The listing builds one solid part. Answer for the finished solid, in the listing's coordinates (mm). A direction names the side the tool comes from. Give positions to 0.01 mm unless a question says otherwise; leave off trailing zeros. Loops run counter-clockwise (first coordinate to the right, second up) from the corner with the lowest first, then second, coordinate; pieces in that order, holes last. Notation, with made-up numbers: (51.25, -21.75) - (69.25, -21.75) arc R14 ccw to (69.25, -10.75) - close; hole circle Ø10 at (85, -10). An arc over 180 degrees is marked (long way). Answer as CSV lines item,"result". Start each with the question number.
1) For faces 1 (the face through (15, 10, -16)), 2 (the face through (18, 9.4, -18)), 3 (the face through (-18, 17, 17)), determine the directions among +Z, -Z, +X, -X, +Y, -Y from which every point of the face is accessible in a straight line to the end or side of a thin tool.
2) Flat-ended cylindrical pins translate along their axes: pin 1 (2.5 mm diameter, centred on x = -15.5, z = -15.5, fed in from +Y); pin 2 (7.5 mm diameter, centred on x = -17, z = 17, fed in from +Y); pin 3 (1.6 mm diameter, centred on x = 15.5, z = 16, fed in from -Y); pin 4 (10 mm diameter, centred on x = -14, y = 41, fed in from -Z). Find the tip coordinate at first contact, or state that the pin passes through.
3) A cutting plane is placed at B-B (z = 0). Determine the outline of the cut face in (x, y).
4) A cutting plane is placed at D-D (y = 20). Determine the outline of the cut face in (x, z), and give its area (3 significant figures).
5) For a pull along Z with two mould halves and no side action, classify faces 4 (the face through (0, 17, -21)), 5 (the face through (-18, 24.6, -18)), 6 (the face through (-15, 29.5, -16)), 7 (the face through (-16, 10, -16)) as pulls with the +Z half, pulls with the -Z half, needs draft (parallel to the pull), parting line crosses it, or undercut.
6) A cutting plane is placed at C-C (x = 0). Determine the outline of the cut face in (y, z).
7) A cutting plane is placed at A-A (y = 5). Determine the outline of the cut face in (x, z).
8) Find the intervals of material crossed by line 1 along X through (y, z) = (6, 15.5); line 2 along X through (y, z) = (34.8, 0); line 3 along Z through (x, y) = (-15, 32), in increasing order.
```python
from build123d import *

# Parameters (mm, degrees)
SKETCH4_W               = 42
SKETCH4_H               = 42
BOTTOM_DEPTH            = 9.4
MIDDLE_DEPTH            = 15.2
SKETCH8_W               = 42
SKETCH8_H               = 42
TOP_DEPTH               = 9.4
CHAMFER1_SIZE           = 5
SKETCH9_R               = 11
SKETCH9_R_2             = 3.5
RING_DEPTH              = 2
SKETCH10_R              = 2.5
SHAFT_DEPTH             = 24
CUT_EXTRUDE3_DEPTH      = 5
CUT_EXTRUDE3_DEPTH_BACK = 5
SKETCH11_W              = 2.239647547
SKETCH11_H              = 24.242457261
SKETCH12_R              = 1.55
CUT_EXTRUDE4_DEPTH      = 4.5
CUT_EXTRUDE5_START      = -10
SKETCH15_R              = 1.55
CUT_EXTRUDE5_DEPTH      = 10


with BuildPart() as part:
    # Sketch4 → Bottom (new body)
    with BuildSketch(Plane(origin=(0, 0, 0), x_dir=(1, 0, 0), z_dir=(0, 1, 0))):
        Rectangle(SKETCH4_W, SKETCH4_H)
    extrude(amount=BOTTOM_DEPTH)

    # Sketch6 → Middle (add)
    with BuildSketch(Plane(origin=(0, 9.4, 0), x_dir=(1, 0, 0), z_dir=(0, 1, 0))):
        Polygon((-21, -14), (-14, -21), (14, -21), (21, -14), (21, 14), (14, 21), (-14, 21), (-21, 14), align=None)
    extrude(amount=MIDDLE_DEPTH)

    # Sketch8 → Top (add)
    with BuildSketch(Plane(origin=(0, 24.6, 0), x_dir=(1, 0, 0), z_dir=(0, 1, 0))):
        Rectangle(SKETCH8_W, SKETCH8_H)
    extrude(amount=TOP_DEPTH)

    # Chamfer1
    chamfer1_edges = [part.edges().sort_by_distance(p)[0] for p in [
        (21, 29.3, 21),
        (21, 29.3, -21),
        (-21, 29.3, -21),
        (-21, 29.3, 21),
        (-21, 4.7, 21),
        (-21, 4.7, -21),
        (21, 4.7, -21),
        (21, 4.7, 21),
    ]]
    chamfer(chamfer1_edges, length=CHAMFER1_SIZE)

    # Sketch9 → Ring (add)
    with BuildSketch(Plane(origin=(0, 34, 0), x_dir=(1, 0, 0), z_dir=(0, 1, 0))):
        with Locations(Location((0, 0, 0), (0, 0, 270))):
            Circle(SKETCH9_R)
        with Locations(Location((0, 0, 0), (0, 0, 270))):
            Circle(SKETCH9_R_2, mode=Mode.SUBTRACT)
    extrude(amount=RING_DEPTH)

    # Sketch10 → Shaft (add)
    with BuildSketch(Plane(origin=(0, 34, 0), x_dir=(1, 0, 0), z_dir=(0, 1, 0))):
        with Locations(Location((0, 0, 0), (0, 0, 90))):
            Circle(SKETCH10_R)
    extrude(amount=SHAFT_DEPTH)

    # Sketch11 → Cut-Extrude3 (cut, two sides: drawn at the far end of the back side and taken through both)
    with BuildSketch(Plane(origin=(0, 0, 0), x_dir=(0, 0, -1), z_dir=(1, 0, 0)).offset(-CUT_EXTRUDE3_DEPTH_BACK)):
        with Locations((2.338622492, 61.12122863)):
            Rectangle(SKETCH11_W, SKETCH11_H)
    extrude(amount=CUT_EXTRUDE3_DEPTH + CUT_EXTRUDE3_DEPTH_BACK, mode=Mode.SUBTRACT)

    # Sketch12 → Cut-Extrude4 (cut)
    with BuildSketch(Plane(origin=(0, 34, 0), x_dir=(1, 0, 0), z_dir=(0, 1, 0))):
        with Locations(Location((15.5, -15.5, 0), (0, 0, 270))):
            Circle(SKETCH12_R)
        with Locations(Location((-15.5, -15.5, 0), (0, 0, 270))):
            Circle(SKETCH12_R)
        with Locations(Location((-15.5, 15.5, 0), (0, 0, 270))):
            Circle(SKETCH12_R)
        with Locations(Location((15.5, 15.5, 0), (0, 0, 270))):
            Circle(SKETCH12_R)
    extrude(amount=-CUT_EXTRUDE4_DEPTH, mode=Mode.SUBTRACT)

    # Sketch15 → Cut-Extrude5 (cut)
    with BuildSketch(Plane.XZ.offset(CUT_EXTRUDE5_START)):
        with Locations(Location((15.5, 15.5, 0), (0, 0, 90))):
            Circle(SKETCH15_R)
        with Locations(Location((15.5, -15.5, 0), (0, 0, 90))):
            Circle(SKETCH15_R)
        with Locations(Location((-15.5, 15.5, 0), (0, 0, 90))):
            Circle(SKETCH15_R)
        with Locations(Location((-15.5, -15.5, 0), (0, 0, 90))):
            Circle(SKETCH15_R)
    extrude(amount=CUT_EXTRUDE5_DEPTH, mode=Mode.SUBTRACT)


solid = part.part
```
Ans:
1,face 1,"-Y"
1,face 2,"-Z, +X"
1,face 3,"+Z, -X"
2,pin 1,"y = 29.5"
2,pin 2,"y = 34"
2,pin 3,"y = 10"
2,pin 4,"through"
3,outline,"(-21, 0) - (21, 0) - (21, 34) - (11, 34) - (11, 36) - (3.5, 36) - (3.5, 34) - (2.5, 34) - (2.5, 58) - (-2.5, 58) - (-2.5, 34) - (-3.5, 34) - (-3.5, 36) - (-11, 36) - (-11, 34) - (-21, 34) - close"
4,outline,"(-21, -14) - (-14, -21) - (14, -21) - (21, -14) - (21, 14) - (14, 21) - (-14, 21) - (-21, 14) - close"
4,area,"1,670 mm2"
5,face 4,"pulls with the -Z half"
5,face 5,"needs draft"
5,face 6,"undercut"
5,face 7,"undercut"
6,outline,"(0, -21) - (34, -21) - (34, -11) - (36, -11) - (36, -3.5) - (34, -3.5) - (34, -2.5) - (49, -2.5) - (49, -1.22) - (58, -1.22) - (58, 2.5) - (34, 2.5) - (34, 3.5) - (36, 3.5) - (36, 11) - (34, 11) - (34, 21) - (0, 21) - close"
7,outline,"(-21, -16) - (-16, -21) - (16, -21) - (21, -16) - (21, 16) - (16, 21) - (-16, 21) - (-21, 16) - close; hole circle Ø3.1 at (-15.5, -15.5); hole circle Ø3.1 at (-15.5, 15.5); hole circle Ø3.1 at (15.5, -15.5); hole circle Ø3.1 at (15.5, 15.5)"
8,line 1,"-21 to -17.05, -13.95 to 13.95, 17.05 to 21"
8,line 2,"-11 to -3.5, -2.5 to 2.5, 3.5 to 11"
8,line 3,"-21 to -16.97, -14.03 to 14.03, 16.97 to 21"
